Work out the finished part from the listing and answer in its coordinate system (mm). Face numbers are marked on the shaded views. A direction names the side the tool comes from. Round coordinates to 2 decimals unless told otherwise and drop trailing zeros. Loops run counter-clockwise (first coordinate to the right, second up) from the corner with the lowest first, then second, coordinate; pieces in that order, holes last. Notation, with made-up numbers: (14, 38.25) -> (53, 38.25) arc R19 ccw to (53, 51.25) -> close; hole circle Ø6 at (67, -2). An arc over 180 degrees is marked (long way). Use one line per item in the form item = value.
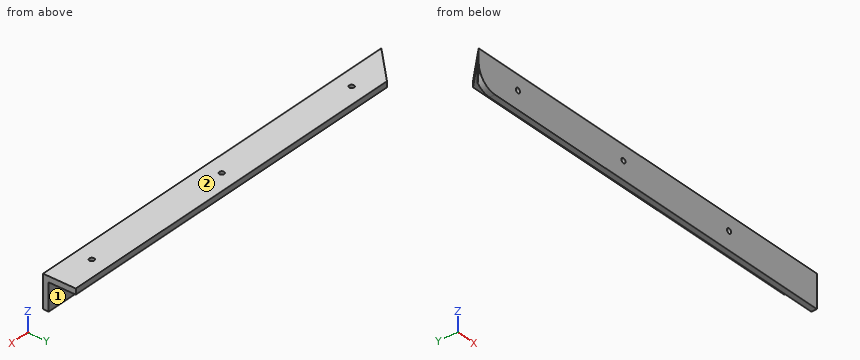
```python
from build123d import *

# Parameters (mm, degrees)
BOSS_EXTRUDE1_DEPTH = 250
SKETCH2_R           = 1.5
CUT_EXTRUDE1_DEPTH  = 252.594912508
SKETCH3_R           = 1.5
CUT_EXTRUDE2_DEPTH  = 252.594912508


with BuildPart() as part:
    # Sketch1 → Boss-Extrude1 (new body)
    with BuildSketch(Plane(origin=(0, 0, 0), x_dir=(0, 0, -1), z_dir=(1, 0, 0))):
        Polygon((0, 0), (20, 0), (20, 3.461178467), (3.461178467, 3.461178467), (3.461178467, 20), (0, 20), align=None)
    extrude(amount=BOSS_EXTRUDE1_DEPTH)

    # Sketch2 → Cut-Extrude1 (cut, through all)
    with BuildSketch(Plane(origin=(0, 0, 0), x_dir=(1, 0, 0), z_dir=(0, 0, -1))):
        with Locations((130, -10)):
            Circle(SKETCH2_R)
        with Locations((34, -10)):
            Circle(SKETCH2_R)
        with Locations((226, -10)):
            Circle(SKETCH2_R)
        Polygon((0, 0), (0, -20), (20, -20), align=None)
    extrude(amount=CUT_EXTRUDE1_DEPTH, mode=Mode.SUBTRACT)

    # Sketch3 → Cut-Extrude2 (cut, through all)
    with BuildSketch(Plane.XZ):
        with Locations(Location((185, -9, 0), (0, 0, 270))):
            Circle(SKETCH3_R)
        with Locations(Location((107, -9, 0), (0, 0, 270))):
            Circle(SKETCH3_R)
        with Locations(Location((29, -9, 0), (0, 0, 270))):
            Circle(SKETCH3_R)
        with BuildLine():
            Line((12, -20), (0, -20))
            Line((0, -20), (0, -8))
            ThreePointArc((0, -8), (3.514718626, -16.485281374), (12, -20))
        make_face()
    extrude(amount=-CUT_EXTRUDE2_DEPTH, mode=Mode.SUBTRACT)


solid = part.part
```
(1) Find section D-D, the plane y = 15. Write down the section's boundary in (x, z).
Completed:
outline = (15, -3.46) -> (250, -3.46) -> (250, 0) -> (15, 0) -> close
(2) Given P1, Ø1, axis at y = 3.5, z = -18, coming from the -X side; P2, Ø5, axis at x = 91.5, y = 13.5, coming from the -Z side; P3, Ø12, axis at y = 8.5, z = -17.5, coming from the -X side; P4, Ø2.5, axis at x = 29, z = -9, coming from the +Y side, each flat-ended and moving along its own axis, determine where each tip first touches the part or whether it passes through.
Completed:
P1 = 4.67
P2 = -3.46
P3 = 2.78
P4 = through
(3) Find section C-C, the plane y = 6. Write down the section's boundary in (x, z).
Completed:
outline = (6, -3.46) -> (250, -3.46) -> (250, 0) -> (6, 0) -> close
(4) Find section A-A, the plane z = -13.5. Write down the section's boundary in (x, y).
Completed:
outline = (1.33, 0) -> (250, 0) -> (250, 3.46) -> (3.46, 3.46) -> (1.33, 1.33) -> close
(5) For the marked faces 1 and 2, determine the directions among +Z, -Z, +X, -X, +Y, -Y from which every point of the face is accessible in a straight line to the end or side of a thin tool.
Completed:
face_1 = -Z, +X, -X, +Y
face_2 = +Z, +X, -X, +Y, -Y
(6) Consider L1, parallel to X at y = 10, z = -2.15; L2, parallel to X at y = 1.35, z = -9; L3, parallel to Z at x = 185, y = 2.75. Determine where each line is inside the solid, lowest interval first.
Completed:
L1 = 10 to 32.5, 35.5 to 128.5, 131.5 to 224.5, 227.5 to 250
L2 = 1.35 to 27.5, 30.5 to 105.5, 108.5 to 183.5, 186.5 to 250
L3 = -20 to -10.5, -7.5 to 0
(7) Find section B-B, the plane x = 99. Write down the section's boundary in (y, z).
Completed:
outline = (0, -20) -> (3.46, -20) -> (3.46, -3.46) -> (20, -3.46) -> (20, 0) -> (0, 0) -> close
